Read the model definition and answer for the solid it produces. Units are mm, in the model's axes. A direction names the side the tool comes from. Give positions to 0.01 mm unless a question says otherwise; leave off trailing zeros. Order: outer loops, then holes, each group sorted by start corner. A loop starts at its lowest first (then second) coordinate and runs counter-clockwise, first axis right, second up.
Autodesk Inventor part; units mm, degrees
ref_plane "YZ Plane" through (0, 0, 0) normal (1, 0, 0) x (0, 1, 0)
ref_plane "XZ Plane" through (0, 0, 0) normal (0, 1, 0) x (-1, 0, 0)
ref_plane "XY Plane" through (0, 0, 0) normal (0, 0, 1) x (1, 0, 0)
sketch "Sketch1" plane through (0, 0, 0) normal (0, 0, 1) x (1, 0, 0)
  circle A0 centre (0, 0) radius 20.32
  circle A1 centre (0, 0) radius 64.77
  circle A2 centre (0, 50.7238) radius 4.8601
  circle A3 centre (-48.2412, 15.6745) radius 4.8601
  circle A4 centre (-29.8147, -41.0364) radius 4.8601
  circle A5 centre (29.8147, -41.0364) radius 4.8601
  circle A6 centre (48.2412, 15.6745) radius 4.8601
  dimension "d0" = 40.64
  dimension "d1" = 129.54
  dimension "d2" = 50.7238
  dimension "d5" = 360
extrude "Extrusion1" add sketch "Sketch1" along normal blind 2.54
sketch "Sketch2" plane through (0, 0, 2.54) normal (0, 0, 1) x (1, 0, 0)
  circle A0 centre (0, 0) radius 20.32
  circle A1 centre (0, 0) radius 20.32
  circle A2 centre (0, 0) radius 64.1368
  circle A3 centre (0, 50.7238) radius 4.8601
  circle A4 centre (0, 50.7238) radius 7.9502
  circle A5 centre (-48.2412, 15.6745) radius 7.9502
  circle A6 centre (-29.8147, -41.0364) radius 7.9502
  circle A7 centre (29.8147, -41.0364) radius 7.9502
  circle A8 centre (48.2412, 15.6745) radius 7.9502
  dimension "d9" = 15.9004
  dimension "d12" = 360
extrude "Extrusion2" add sketch "Sketch2" along normal blind 2.54 contours A2
properties part number "Savior Paddle Template"
1) Given pin 1 (1 mm diameter, centred on y = -41.5, z = 2.5, fed in from -X); pin 2 (14.5 mm diameter, centred on x = 29.81, y = -41.04, fed in from +Z); pin 3 (3 mm diameter, centred on x = -6.5, z = 2.5, fed in from -Y), each flat-ended and moving along its own axis, determine where each tip first touches the part or whether it passes through.
Final values:
pin 1: stops at x = -50.14
pin 2: stops at z = 2.54
pin 3: stops at y = -64.58
2) The part is cut by section B-B on y = 0. Determine the outline of the cut face in (x, z).
Final values:
outline: (-64.77, 0) - (-20.32, 0) - (-20.32, 5.08) - (-64.14, 5.08) - (-64.14, 2.54) - (-64.77, 2.54) - close; (20.32, 0) - (64.77, 0) - (64.77, 2.54) - (64.14, 2.54) - (64.14, 5.08) - (20.32, 5.08) - close
3) The part is cut by section C-C on z = 3.85. Determine the outline of the cut face in (x, y).
Final values:
outline: circle Ø128.27 at (0, 0); hole circle Ø15.9 at (-48.24, 15.67); hole circle Ø15.9 at (-29.81, -41.04); hole circle Ø40.64 at (0, 0); hole circle Ø15.9 at (0, 50.72); hole circle Ø15.9 at (29.81, -41.04); hole circle Ø15.9 at (48.24, 15.67)
4) Consider L1, parallel to X at y = -42.5, z = 1.1; L2, parallel to Z at x = 3.5, y = 46; L3, parallel to Y at x = 11.5, z = 2.5. Determine where each line is inside the solid, lowest interval first.
Final values:
L1: x = -48.88 to -34.45, -25.18 to 25.18, 34.45 to 48.88
L2: z = 0 to 2.54
L3: y = -63.74 to -16.75, 16.75 to 63.74
5) A tool of negligible diameter and unlimited length cuts with its end or side. For faces 5 (the face through (-22.23, -43.42, 3.79)), 6 (the face through (-2.645, -20.147, 2.504)), from which of +Z, -Z, +X, -X, +Y, -Y can it reach the whole face along a straight path? Write none if from no direction.
Final values:
face 5: +Z
face 6: +Z, -Z
6) The part is cut by section A-A on x = 0. Determine the outline of the cut face in (y, z), and give its area (3 significant figures).
Final values:
outline: (-64.77, 0) - (-20.32, 0) - (-20.32, 5.08) - (-64.14, 5.08) - (-64.14, 2.54) - (-64.77, 2.54) - close; (20.32, 0) - (45.86, 0) - (45.86, 2.54) - (42.77, 2.54) - (42.77, 5.08) - (20.32, 5.08) - close; (55.58, 0) - (64.77, 0) - (64.77, 2.54) - (64.14, 2.54) - (64.14, 5.08) - (58.67, 5.08) - (58.67, 2.54) - (55.58, 2.54) - close
area: 383 mm2
7) The part is cut by section D-D on x = -13. Determine the outline of the cut face in (y, z).
Final values:
outline: (-63.45, 0) - (-15.62, 0) - (-15.62, 5.08) - (-62.81, 5.08) - (-62.81, 2.54) - (-63.45, 2.54) - close; (15.62, 0) - (63.45, 0) - (63.45, 2.54) - (62.81, 2.54) - (62.81, 5.08) - (15.62, 5.08) - close
8) For a pull along Y with two mould halves and no side action, classify faces 1 (the face through (-40.658, 13.286, 3.792)), 2 (the face through (-15, 15, 5.08)), 3 (the face through (-8.35, -63.59, 3.79)), 4 (the face through (-52.1, 18.63, 1.25)) as released by +Y, released by -Y, zero draft, split by the parting line, or undercut.
Final values:
face 1: undercut
face 2: zero draft
face 3: split by the parting line
face 4: undercut
